Read the model definition and answer for the solid it produces. Units are mm, in the model's axes. A direction names the side the tool comes from. Give positions to 0.01 mm unless a question says otherwise; leave off trailing zeros. Order: outer loops, then holes, each group sorted by start corner. A loop starts at its lowest first (then second) coordinate and runs counter-clockwise, first axis right, second up.
Item 1: A cutting plane is placed at A-A (x = 1). Write down the section's boundary in (y, z), plus the area to 3 significant figures.
Item 2: A cutting plane is placed at C-C (y = -7.5). Write down the section's boundary in (x, z), plus the area to 3 significant figures.
Item 3: Given pin 1 Ø1.5 at (y, z) = (-9, -1.5) entering from +X; pin 2 Ø3 at (y, z) = (-10, -6) entering from +X; pin 3 Ø6 at (y, z) = (-2.5, 8) entering from +X, each flat-ended and moving along its own axis, determine where each tip first touches the part or whether it passes through.
Item 4: A cutting plane is placed at D-D (y = -20.25). Write down the section's boundary in (x, z) (1 decimal).
Item 5: Which of the six approach directions +Z, -Z, +X, -X, +Y, -Y give full straight-line access (tool end or side, diameter ignored) to faces 4 (the face through (5, -25.4, 0)), 5 (the face through (4.762, -5, 0))?
Item 6: Find the intervals of material crossed by line 1 along Z through (x, y) = (-4.5, -2); line 2 along X through (y, z) = (-12.25, -1.75); line 3 along Z through (x, y) = (3.5, -5), in increasing order.
Item 7: The mould has two halves that part along X. Classify faces 1 (the face through (5, 0, 0)), 2 (the face through (-2.75, -12.52, -12.4)), 3 (the face through (0, -5, -4.762)): +X half, -X half, draft (parallel to the pull), parting line (faces both ways), or undercut.
from build123d import *

# Parameters (mm, degrees)
F0_R      = 12.7
F1_DEPTH  = 25.4
F1_FACE_R = 12.7
F3_DEPTH  = 25.4
F4_DEPTH  = 25.401
F5_DEPTH  = 11.0998


with BuildPart() as f1:
    # F0 (on Front) → F1 (new body)
    with BuildSketch(Plane.XZ):
        Circle(F0_R)
    extrude(amount=F1_DEPTH)

    # F1_face (on face) → F3 (cut)
    with BuildSketch(Plane.XZ.offset(25.4)):
        Circle(F1_FACE_R)
    extrude(amount=F3_DEPTH, mode=Mode.SUBTRACT)

    # F2 (on Front) → F4 (cut, through all)
    with BuildSketch(Plane.XZ):
        with BuildLine():
            ThreePointArc((4.7625, 0), (3.367596, 3.367596), (0, 4.7625))
            ThreePointArc((0, 4.7625), (-3.367596, 3.367596), (-4.7625, 0))
            ThreePointArc((-4.7625, 0), (-3.367596, -3.367596), (0, -4.7625))
            ThreePointArc((0, -4.7625), (3.367596, -3.367596), (4.7625, 0))
        make_face()
    extrude(amount=F4_DEPTH, mode=Mode.SUBTRACT)

    # F2 (on Front) → F5 (cut)
    with BuildSketch(Plane.XZ):
        with BuildLine():
            Line((4.7625, 0), (4.7625, 4.7625))
            Line((4.7625, 4.7625), (0, 4.7625))
            ThreePointArc((0, 4.7625), (3.367596, 3.367596), (4.7625, 0))
        make_face()
        with BuildLine():
            ThreePointArc((-4.7625, 0), (-3.367596, 3.367596), (0, 4.7625))
            Line((0, 4.7625), (-4.7625, 4.7625))
            Line((-4.7625, 4.7625), (-4.7625, 0))
        make_face()
        with BuildLine():
            Line((4.7625, -4.7625), (4.7625, 0))
            ThreePointArc((4.7625, 0), (3.367596, -3.367596), (0, -4.7625))
            Line((0, -4.7625), (4.7625, -4.7625))
        make_face()
        with BuildLine():
            ThreePointArc((0, -4.7625), (-3.367596, -3.367596), (-4.7625, 0))
            Line((-4.7625, 0), (-4.7625, -4.7625))
            Line((-4.7625, -4.7625), (0, -4.7625))
        make_face()
    extrude(amount=F5_DEPTH, mode=Mode.SUBTRACT)


solid = f1.part
Response values:
1. outline: (-25.4, -12.66) - (0, -12.66) - (0, -4.76) - (-11.1, -4.76) - (-11.1, -4.66) - (-25.4, -4.66) - close; (-25.4, 4.66) - (-11.1, 4.66) - (-11.1, 4.76) - (0, 4.76) - (0, 12.66) - (-25.4, 12.66) - close
1. area: 404 mm2
2. outline: circle Ø25.4 at (0, 0); hole (-4.76, -4.76) - (4.76, -4.76) - (4.76, 4.76) - (-4.76, 4.76) - close
2. area: 416 mm2
3. pin 1: stops at x = 12.68
3. pin 2: stops at x = 11.88
3. pin 3: stops at x = 11.67
4. outline: circle Ø25.4 at (0, 0); hole circle Ø9.5 at (0, 0)
5. face 4: +Z, -Z, +X, -X, -Y
5. face 5: +Y
6. line 1: z = -11.88 to -4.76, 4.76 to 11.88
6. line 2: x = -12.58 to -4.43, 4.43 to 12.58
6. line 3: z = -12.21 to -4.76, 4.76 to 12.21
7. face 1: draft
7. face 2: parting line
7. face 3: undercut
